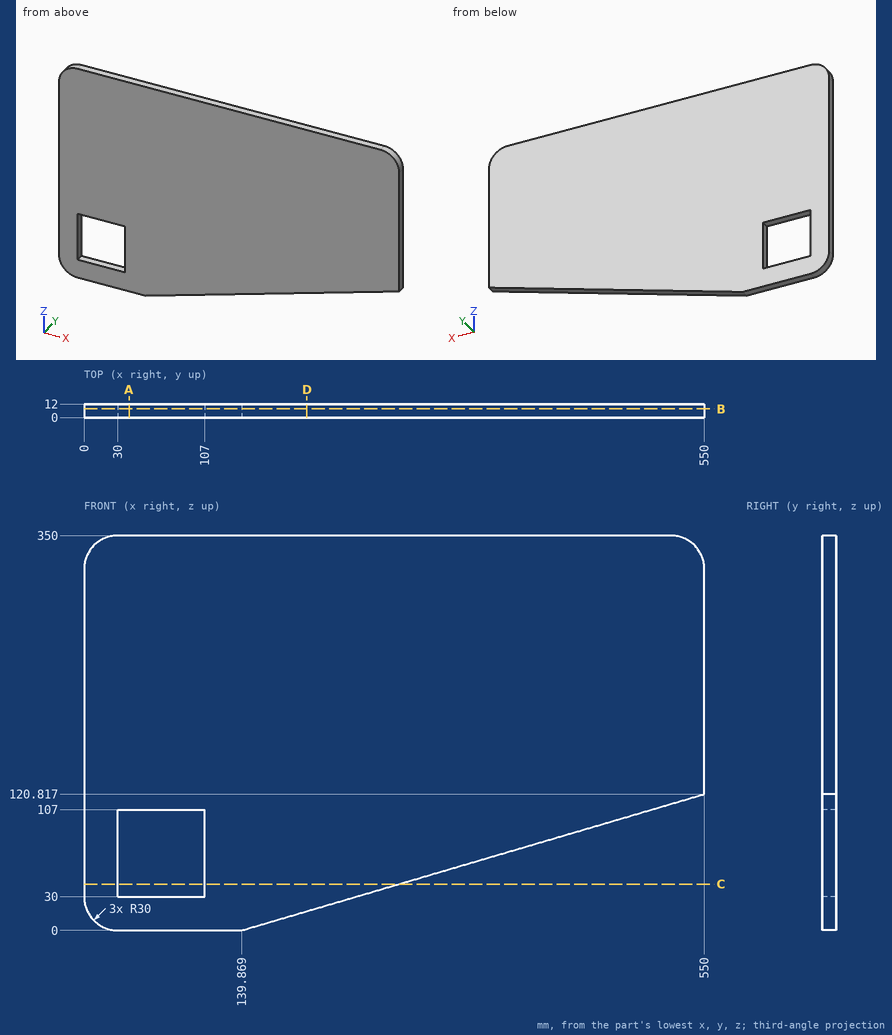
Here's the drawing with two shaded views (mm, measured from the low corner). I have some questions. Give positions to 0.01 mm unless a question says otherwise; leave off trailing zeros. Write each loop counter-clockwise with the first axis right and the second up, starting at its lowest first coordinate (ties: lowest second). Pieces come first, ordered by that corner, then holes. Notation, with made-up numbers: (-17, 7) - (28, 7) arc R17 cw to (28, 29) - close; hole circle Ø7 at (-6.75, 19). An arc over 180 degrees is marked (long way). Write item = value, one per line. Start each with the question number.
1. For pin 1 (2 mm diameter, centred on x = 164, z = 299.5, fed in from -Y), with a flat end and sliding along its axis, tell me the tip position at first contact or that it passes through.
2. Imagine slicing it at C-C (z = 41). Please give me the cut outline in (x, y).
3. Please list where these lines run through material, in increasing order: line 1 (Z direction, x = 48, y = 8.25); line 2 (Z direction, x = 489.5, y = 10.5) (1 decimal); line 3 (Z direction, x = 517, y = 7) (1 decimal).
4. Imagine slicing it at B-B (y = 7.75). Please give me the cut outline in (x, z), and give its area (3 significant figures).
5. Imagine slicing it at D-D (x = 197.5). Please give me the cut outline in (y, z), and give its area (3 significant figures).
6. Imagine slicing it at A-A (x = 40). Please give me the cut outline in (y, z), and give its area (3 significant figures).
Worked answers:
q1.pin_1 = 0
q2.outline = (0, 0) - (30, 0) - (30, 12) - (0, 12) - close; (107, 0) - (279.05, 0) - (279.05, 12) - (107, 12) - close
q3.line_1 = 0 to 30, 107 to 350
q3.line_2 = 103 to 350
q3.line_3 = 111.1 to 350
q4.outline = (0, 30) arc R30 ccw to (30, 0) - (139.87, 0) - (550, 120.82) - (550, 320) arc R30 ccw to (520, 350) - (30, 350) arc R30 ccw to (0, 320) - close; hole (30, 30) - (107, 30) - (107, 107) - (30, 107) - close
q4.area = 161,000 mm2
q5.outline = (0, 16.98) - (12, 16.98) - (12, 350) - (0, 350) - close
q5.area = 4,000 mm2
q6.outline = (0, 0) - (12, 0) - (12, 30) - (0, 30) - close; (0, 107) - (12, 107) - (12, 350) - (0, 350) - close
q6.area = 3,280 mm2
